Build history of the part. All positions in model axes, mm. A direction names the side the tool comes from. Round coordinates to 2 decimals unless told otherwise and drop trailing zeros. Order: outer loops, then holes, each group sorted by start corner. A loop starts at its lowest first (then second) coordinate and runs counter-clockwise, first axis right, second up. Notation, with made-up numbers: M -25.75,-20.75 L 23.25,-20.75 A32 ccw 23.25,6.25 Z; hole C 12.5,21 d11. An arc over 180 degrees is marked long. Use CSV: the item, a comma, the result in double quotes.
from build123d import *

# Parameters (mm, degrees)
F0_R      = 12
F1_DEPTH  = 30.5
F2_R      = 1
F3_DEPTH  = 11.5
F4_R      = 3.175
F5_DEPTH  = 1.6
F6_R      = 1.3
F7_DEPTH  = 10
F8_R      = 4
F9_DEPTH  = 2
F10_W     = 0.5
F10_H     = 3
F11_DEPTH = 5.2
F12_R     = 1
F13_R     = 1
F14_R     = 1


with BuildPart() as f1:
    # F0 (on Top) → F1 (new body)
    with BuildSketch(Plane.XY):
        Circle(F0_R)
    extrude(amount=F1_DEPTH)

    # F2 (on face) → F3 (join)
    with BuildSketch(Plane.XY.offset(30.5)):
        Circle(F2_R)
    extrude(amount=F3_DEPTH)

    # F4 (on face) → F5 (join)
    with BuildSketch(Plane.XY.offset(30.5)):
        Circle(F4_R)
    extrude(amount=F5_DEPTH)

    # F6 (on face) → F7 (cut)
    with BuildSketch(Plane.XY.offset(30.5)):
        with Locations((-7, 0)):
            Circle(F6_R)
        with Locations((7, 0)):
            Circle(F6_R)
    extrude(amount=-F7_DEPTH, mode=Mode.SUBTRACT)

    # F8 (on face) → F9 (join)
    with BuildSketch(Plane(origin=(0, 0, 0), x_dir=(1, 0, 0), z_dir=(0, 0, -1))):
        Circle(F8_R)
    extrude(amount=F9_DEPTH)

    # F10 (on face) → F11 (join)
    with BuildSketch(Plane(origin=(0, 0, 0), x_dir=(1, 0, 0), z_dir=(0, 0, -1))):
        with Locations((-9.45, 0)):
            Rectangle(F10_W, F10_H)
        with Locations((9.45, 0)):
            Rectangle(F10_W, F10_H)
    extrude(amount=F11_DEPTH)

    # F12
    f12_edges = [f1.edges().sort_by_distance(p)[0] for p in [
        (-9.45, 1.5, -5.2),
        (-9.45, -1.5, -5.2),
        (9.45, 1.5, -5.2),
        (9.45, -1.5, -5.2),
    ]]
    fillet(f12_edges, radius=F12_R)

    # F13
    f13_edges = [f1.edges().sort_by_distance(p)[0] for p in [
        (-12, 0, 0),
    ]]
    fillet(f13_edges, radius=F13_R)

    # F14
    f14_edges = [f1.edges().sort_by_distance(p)[0] for p in [
        (-12, 0, 30.5),
    ]]
    fillet(f14_edges, radius=F14_R)


solid = f1.part
(1) Drop flat-ended pins along their axis: pin 1 (1.3 mm diameter, centred on x = -7.5, y = 0, fed in from +Z); pin 2 (1.5 mm diameter, centred on y = 0, z = -3, fed in from +X); pin 3 (3.5 mm diameter, centred on x = 7, y = 0, fed in from -Z); pin 4 (12 mm diameter, centred on x = 6, y = -1, fed in from +Z). Give the stop position or say it passes through.
Answer block:
pin 1,"stops at z = 20.5"
pin 2,"stops at x = 9.7"
pin 3,"stops at z = 0"
pin 4,"stops at z = 42"
(2) Tool access for faces 1 (the face through (-9.7, 0, -3)), 2 (the face through (9.7, 0, -3)), 3 (the face through (-9.2, 0, -3)), 4 (the face through (-0.867, 3.905, -0.986)), 5 (the face through (-5.76, 0.39, 25.57)): list every direction of +Z, -Z, +X, -X, +Y, -Y with a clear straight run to the whole face (end or side of a thin tool).
Answer block:
face 1,"-Z, -X, +Y, -Y"
face 2,"-Z, +X, +Y, -Y"
face 3,"-Z, +Y, -Y"
face 4,"-Z"
face 5,"+Z"
(3) Cut at A-A, the plane x = 0. Give the cut face in (y, z) (3 decimals).
Answer block:
outline,"M -12,1 A1 ccw -11,0 L -4,0 L -4,-2 L 4,-2 L 4,0 L 11,0 A1 ccw 12,1 L 12,29.5 A1 ccw 11,30.5 L 3.175,30.5 L 3.175,32.1 L 1,32.1 L 1,42 L -1,42 L -1,32.1 L -3.175,32.1 L -3.175,30.5 L -11,30.5 A1 ccw -12,29.5 Z"
(4) Cut at B-B, the plane z = 13.5. Give the cut face in (x, y), and give its area (3 significant figures).
Answer block:
outline,"C 0,0 d24"
area,"452 mm²"
(5) Wall check: line 1 (Z direction, x = 8, y = 1.5); line 2 (Y direction, x = 7, z = 28); line 3 (Z direction, x = 1, y = -2.75). Give the ranges that are in metal, low to high. Write a range as from..to.
Answer block:
line 1,"z = 0..30.5"
line 2,"y = -9.75..-1.3, 1.3..9.75"
line 3,"z = -2..32.1"
(6) Cut at C-C, the plane z = 37. Give the cut face in (x, y).
Answer block:
outline,"C 0,0 d2"
